Design review of the part built by this model. Coordinates are the model's own, in mm. A direction names the side the tool comes from. Give positions to 0.01 mm unless a question says otherwise; leave off trailing zeros. Use CSV: the item, a comma, the result in double quotes.
```python
from build123d import *

# Parameters (mm, degrees)
F4_R     = 2.5
F5_DEPTH = 25


with BuildPart() as f1:
    # F0 (on Front) → F1 (revolve)
    with BuildSketch(Plane.XZ):
        with BuildLine():
            Line((0, 39), (0, 0))
            Line((0, 0), (21, 0))
            Line((21, 0), (21, 42))
            Line((21, 42), (14.571175, 42))
            Line((14.571175, 42), (13.965926, 39.741181))
            ThreePointArc((13.965926, 39.741181), (13, 39), (12.034074, 39.741181))
            Line((12.034074, 39.741181), (10.223054, 46.5))
            Line((10.223054, 46.5), (6, 46.5))
            Line((6, 46.5), (3.990381, 39))
            Line((3.990381, 39), (0, 39))
        make_face()
    revolve(axis=Axis((10.5, 0, 0), (-1, 0, 0)))

    # F2 (on Front) → F3 (revolve, cut)
    with BuildSketch(Plane.XZ):
        Polygon((0, 28.5), (0, 0), (24, 0), (24, 28.5), (18, 28.5), (18, 21), (11.96849, 21), (9.238713, 28.5), align=None)
    revolve(axis=Axis((12, 0, 0), (-1, 0, 0)), mode=Mode.SUBTRACT)

    # F4 (on Right) → F5 (cut)
    with BuildSketch(Plane.YZ):
        with Locations((-35.390936, 0)):
            Circle(F4_R)
        with Locations((-30.649449, -17.695468)):
            Circle(F4_R)
        with Locations((-17.695468, -30.649449)):
            Circle(F4_R)
        with Locations((0, -35.390936)):
            Circle(F4_R)
        with Locations((17.695468, -30.649449)):
            Circle(F4_R)
        with Locations((30.649449, -17.695468)):
            Circle(F4_R)
        with Locations((35.390936, 0)):
            Circle(F4_R)
        with Locations((30.649449, 17.695468)):
            Circle(F4_R)
        with Locations((17.695468, 30.649449)):
            Circle(F4_R)
        with Locations((0, 35.390936)):
            Circle(F4_R)
        with Locations((-17.695468, 30.649449)):
            Circle(F4_R)
        with Locations((-30.649449, 17.695468)):
            Circle(F4_R)
    extrude(amount=F5_DEPTH, mode=Mode.SUBTRACT)


solid = f1.part
```
(1) Clearance check with flat-ended pins moving along their axes: pin 1 (2 mm diameter, centred on x = 9, y = 11.5, fed in from +Z); pin 2 (3 mm diameter, centred on x = 18.5, y = 33, fed in from -Z); pin 3 (10 mm diameter, centred on x = 6.5, z = -5, fed in from -Y). State where each tip first meets the part, or that it passes through.
Established:
pin 1,"stops at z = 45.3"
pin 2,"stops at z = -27.78"
pin 3,"stops at y = -46.5"
(2) Mouldability with a two-part tool opening along Y and no side actions: class faces 4 (the face through (10.353, -16.351, -28.541)), 5 (the face through (21, 29, 1)), 6 (the face through (8.08, 13.97, 44.35)) as +Y half, -Y half, draft (parallel to the pull), parting line (faces both ways), or undercut.
Established:
face 4,"undercut"
face 5,"draft"
face 6,"parting line"
(3) For line 1 along Y through (x, z) = (2.25, 0.5); line 2 along Z through (x, y) = (8, -17); line 3 along Y through (x, z) = (18.75, 0), list the stretches that pass through material, from the lowest coordinate up. Write a range as [from, to].
Established:
line 1,"y = [-39, -37.84], [-32.94, -28.5], [28.5, 32.94], [37.84, 39]"
line 2,"z = [-43.28, -33.05], [-28.25, -22.87], [22.87, 28.25], [33.05, 43.28]"
line 3,"y = [-42, -37.89], [-32.89, -28.5], [28.5, 32.89], [37.89, 42]"
(4) Take a section at A-A (y = 0). State how many separate pieces and enclosed holes the cut face has, then the cut area to 3 significant figures.
Established:
separate pieces,"4"
enclosed holes,"0"
area,"477 mm2"
(5) Tool access review of faces 1 (the face through (11.92, -39.21, -8.71)), 2 (the face through (4.555, -10.916, 26.327)), 3 (the face through (19.479, -10.916, 26.327)): name each direction out of +Z, -Z, +X, -X, +Y, -Y from which nothing blocks a thin tool from reaching the whole face with its end or side.
Established:
face 1,"none"
face 2,"-X"
face 3,"+X"
